```python
from build123d import *

# Parameters (mm, degrees)
SKETCH010_R                = 3.5
EXTRUDE009_DEPTH           = 6
FILLET001_R                = 2
EXTRUDE023_DEPTH           = 75
EXTRUDE023_PLACEMENT_ANGLE = 180


with BuildPart() as obj1:
    # Sketch010 → Extrude009 (new body)
    with BuildSketch(Plane(origin=(0, 0, 0), x_dir=(0, -1, 0), z_dir=(-1, 0, 0))):
        with BuildLine():
            ThreePointArc((0, 7.5), (-7.5, 0), (0, -7.5))
            Line((0, -7.5), (90, -7.5))
            ThreePointArc((90, -7.5), (97.5, 0), (90, 7.5))
            Line((0, 7.5), (90, 7.5))
        make_face()
        Circle(SKETCH010_R, mode=Mode.SUBTRACT)
        with Locations((90, 0)):
            Circle(SKETCH010_R, mode=Mode.SUBTRACT)
    extrude(amount=EXTRUDE009_DEPTH)


with BuildPart() as obj1_1:
    # Extrude009 placement: moved
    add(obj1.part.moved(Location((60, 5.35, 173.65))))

    # Fillet001
    fillet001_edges = [obj1_1.edges().sort_by_distance(p)[0] for p in [
        (54, -39.65, 181.15),
    ]]
    fillet(fillet001_edges, radius=FILLET001_R)


with BuildPart() as fusion028:
    # Sketch024 → Extrude023 (new body)
    with BuildSketch(Plane.XZ):
        with BuildLine():
            ThreePointArc((-4.21383, -5.589601), (7, 0), (-4.21383, 5.589601))
            ThreePointArc((-4.21383, -5.589601), (3.372719, 0), (-4.21383, 5.589601))
        make_face()
    extrude(amount=EXTRUDE023_DEPTH)


with BuildPart() as fusion028_1:
    # Extrude023 placement: moved
    add(fusion028.part.moved(Location((53.5, -5, 173.6))).rotate(Axis((53.5, -5, 173.6), (0, 1, 0)), EXTRUDE023_PLACEMENT_ANGLE))

    # Fusion028: union obj1
    add(obj1_1.part)


with BuildPart() as fusion028_2:
    # Fusion028 placement: moved
    add(fusion028_1.part.moved(Location((-4, 0, 0))))


solid = fusion028_2.part
```
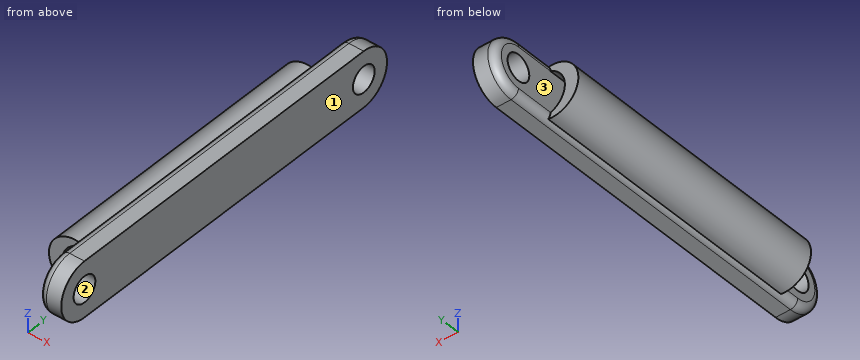
The listing builds one solid part. Answer for the finished solid, in the listing's coordinates (mm). Face numbers are marked on the shaded views. Coordinates: 2 decimals unless noted, no trailing zeros. Loops run counter-clockwise (first coordinate to the right, second up) from the corner with the lowest first, then second, coordinate; pieces in that order, holes last. Notation, with made-up numbers: (-21, 43) - (1, 43) arc R16 ccw to (1, 72) - close; hole circle Ø1 at (84, -0.75). An arc over 180 degrees is marked (long way). Write item = value, one per line.
1) Each of these flat-tipped pins is pushed along its axis until it touches: P1, Ø4, axis at x = 45.5, z = 172, coming from the +Y side; P2, Ø6, axis at x = 45, y = -17, coming from the -Z side; P3, Ø8, axis at y = -45, z = 178, coming from the -X side. Where does it stop, or does it pass through?
Responses:
P1 = -5
P2 = 166.76
P3 = 42.51
2) Section C-C (z = 173.65) is taken. Determine the outline of the cut face in (x, y).
Responses:
outline = (42.5, -80) - (46.13, -80) - (46.13, -5) - (42.5, -5) - close; (50, -90.15) arc R2 ccw to (52, -92.15) - (56, -92.15) - (56, -88.15) - (50, -88.15) - close; (50, -81.15) - (56, -81.15) - (56, 1.85) - (50, 1.85) - close; (50, 8.85) - (56, 8.85) - (56, 12.85) - (52, 12.85) arc R2 ccw to (50, 10.85) - close
3) Determine the mould class of the marked faces 1, 2 and 3 for opening direction X: pulls with the +X half, pulls with the -X half, needs draft (parallel to the pull), parting line crosses it, or undercut.
Responses:
face_1 = pulls with the +X half
face_2 = needs draft
face_3 = undercut
4) Section A-A (x = 54.5) is taken. Determine the outline of the cut face in (y, z), plus the area to 3 significant figures.
Responses:
outline = (-84.65, 166.15) - (5.35, 166.15) arc R7.5 ccw to (5.35, 181.15) - (-84.65, 181.15) arc R7.5 ccw to start; hole circle Ø7 at (-84.65, 173.65); hole circle Ø7 at (5.35, 173.65)
area = 1,450 mm^2
5) Section D-D (y = -65.5) is taken. Determine the outline of the cut face in (x, z), plus the area to 3 significant figures.
Responses:
outline = (50.54, 180.52) arc R7 ccw (long way) to (50.63, 166.69) arc R2 ccw to (52, 166.15) - (56, 166.15) - (56, 181.15) - (52, 181.15) arc R2 ccw to start; hole (50, 168.09) arc R2 cw to (50, 168.15) - (50, 179.11) arc R5.85 ccw to start
area = 142 mm^2
6) Find the intervals of material crossed by line 1 along Y through (x, z) = (53.5, 173.65); line 2 along Y through (x, z) = (52.5, 176.5); line 3 along X through (y, z) = (-73, 174), in increasing order.
Responses:
line_1 = -92.15 to -88.15, -81.15 to 1.85, 8.85 to 12.85
line_2 = -91.59 to -86.68, -82.62 to 3.32, 7.38 to 12.29
line_3 = 42.51 to 46.14, 50 to 56
7) Section B-B (y = 3.5) is taken. Determine the outline of the cut face in (x, z).
Responses:
outline = (50, 168.15) arc R2 ccw to (52, 166.15) - (56, 166.15) - (56, 170.68) - (50, 170.68) - close; (50, 176.62) - (56, 176.62) - (56, 181.15) - (52, 181.15) arc R2 ccw to (50, 179.15) - close
